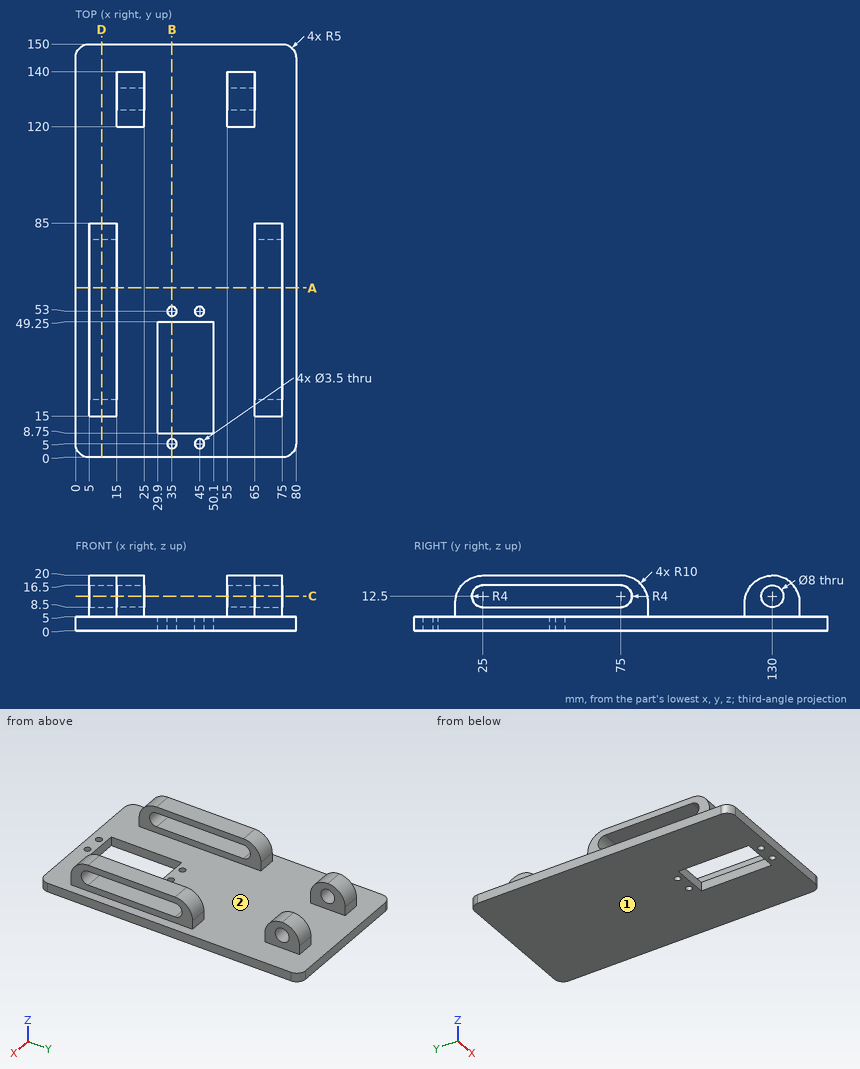
Job drawing, mm, ordinate dimensions from the low corner. One solid piece. Give positions to 0.01 mm unless a question says otherwise; leave off trailing zeros. Order: outer loops, then holes, each group sorted by start corner. A loop starts at its lowest first (then second) coordinate and runs counter-clockwise, first axis right, second up. Notation, with made-up numbers: M -30,24 L -9,24 A28 ccw -9,50 Z; hole C -17,74 d5. An arc over 180 degrees is marked long. Return JSON: item names as keys, results as strings.
Q1. Two-plate mould, pull along X, no slides. Class the marked faces 1 and 2: pulls with the +X half, pulls with the -X half, needs draft (parallel to the pull), parting line crosses it, or undercut.
Answer list:
{"face 1": "needs draft", "face 2": "undercut"}
Q2. Band-saw the part on A-A (y = 61.5). Give the cut face in (x, z), then the cut area to 3 significant figures.
Answer list:
{"outline": "M 0,0 L 80,0 L 80,5 L 75,5 L 75,8.5 L 65,8.5 L 65,5 L 15,5 L 15,8.5 L 5,8.5 L 5,5 L 0,5 Z; M 5,16.5 L 15,16.5 L 15,20 L 5,20 Z; M 65,16.5 L 75,16.5 L 75,20 L 65,20 Z", "area": "540 mm^2"}
Q3. Band-saw the part on C-C (z = 12.5). Count the separate pieces of the cut face and the enclosed holes in it, then the cut area to 3 significant figures.
Answer list:
{"separate pieces": "8", "enclosed holes": "0", "area": "455 mm^2"}
Q4. Wall check: probe 1 along Y at (x, z) = (45, 3.8); probe 2 along X at (y, z) = (53, 2.45); probe 3 along X at (y, z) = (43.5, 3). Give the ranges that are in metal, low to high. Write a range as from..to.
Answer list:
{"probe 1": "y = 0..3.25, 6.75..8.75, 49.25..51.25, 54.75..150", "probe 2": "x = 0..33.25, 36.75..43.25, 46.75..80", "probe 3": "x = 0..29.9, 50.1..80"}
Q5. Band-saw the part on D-D (x = 9.5). Give the cut face in (y, z), then the cut area to 3 significant figures.
Answer list:
{"outline": "M 0,0 L 150,0 L 150,5 L 85,5 L 85,10 A10 ccw 75,20 L 25,20 A10 ccw 15,10 L 15,5 L 0,5 Z; hole M 25,8.5 L 75,8.5 A4 ccw 75,16.5 L 25,16.5 A4 ccw Z", "area": "1,310 mm^2"}
Q6. Band-saw the part on B-B (x = 35). Give the cut face in (y, z).
Answer list:
{"outline": "M 0,0 L 3.25,0 L 3.25,5 L 0,5 Z; M 6.75,0 L 8.75,0 L 8.75,5 L 6.75,5 Z; M 49.25,0 L 51.25,0 L 51.25,5 L 49.25,5 Z; M 54.75,0 L 150,0 L 150,5 L 54.75,5 Z"}
Q7. Flat gauge pins, fed straight in: pin 1 (4 mm diameter, centred on x = 69.5, z = 8.5, fed in from +Y); pin 2 (4 mm diameter, centred on x = 58, z = 7.5, fed in from +Y); pin 3 (5.5 mm diameter, centred on x = 35, y = 53, fed in from +Z). Where does each tip first touch, or does it go through?
Answer list:
{"pin 1": "stops at y = 85", "pin 2": "stops at y = 140", "pin 3": "stops at z = 5"}
